from build123d import *

# Parameters (mm, degrees)
SKETCH_R     = 2.25
SKETCH_R_2   = 11.25
SKETCH_R_3   = 1.75
PAD_DEPTH    = 12
POCKET_DEPTH = 9


with BuildPart() as pocket_belt_path:
    # Sketch → Pad (new body)
    with BuildSketch(Plane.XY):
        Polygon((0, 0), (105, 0), (105, 62), (20, 62), (20, 42), (0, 42), align=None)
        with Locations((35, 10)):
            Circle(SKETCH_R, mode=Mode.SUBTRACT)
        with Locations((30, 35)):
            Circle(SKETCH_R, mode=Mode.SUBTRACT)
        with Locations((84, 21)):
            Circle(SKETCH_R_2, mode=Mode.SUBTRACT)
        with Locations((68.5, 36.5)):
            Circle(SKETCH_R_3, mode=Mode.SUBTRACT)
        with Locations((99.5, 36.5)):
            Circle(SKETCH_R_3, mode=Mode.SUBTRACT)
        with Locations((68.5, 5.5)):
            Circle(SKETCH_R_3, mode=Mode.SUBTRACT)
        with Locations((99.5, 5.5)):
            Circle(SKETCH_R_3, mode=Mode.SUBTRACT)
        with Locations((10, 30)):
            Circle(SKETCH_R, mode=Mode.SUBTRACT)
        with Locations((10, 15)):
            Circle(SKETCH_R, mode=Mode.SUBTRACT)
        with Locations((39, 52)):
            Circle(SKETCH_R, mode=Mode.SUBTRACT)
        with Locations((94, 52)):
            Circle(SKETCH_R, mode=Mode.SUBTRACT)
        with Locations((55, 5)):
            Circle(SKETCH_R, mode=Mode.SUBTRACT)
        with BuildLine():
            Line((58.75, 25), (58.75, 40))
            ThreePointArc((58.75, 40), (56.5, 42.25), (54.25, 40))
            Line((54.25, 25), (54.25, 40))
            ThreePointArc((54.25, 25), (56.5, 22.75), (58.75, 25))
        make_face(mode=Mode.SUBTRACT)
    extrude(amount=PAD_DEPTH)

    # Sketch001 → Pocket (cut)
    with BuildSketch(Plane.XY.offset(12)):
        with BuildLine():
            ThreePointArc((38.485281, 42), (36.015595, 44.209377), (32.999996, 45.583006))
            Line((32.999996, 67), (32.999996, 45.583006))
            Line((20, 67), (32.999996, 67))
            Line((20, -1), (20, 67))
            Line((20, -1), (48.252269, -1))
            Line((48.252269, 11), (48.252269, -1))
            Line((48.252269, 11), (70.252269, 11))
            ThreePointArc((70.252269, 11), (71.759618, 9.202833), (73.499996, 7.630258))
            Line((73.499996, 7.630258), (73.499996, -1))
            Line((73.499996, -1), (93.499996, -1))
            Line((93.499996, -1), (93.499996, 6.902128))
            ThreePointArc((93.499996, 6.902128), (95.574295, 8.548671), (97.367695, 10.497399))
            Line((105.499996, 10.497399), (97.367695, 10.497399))
            Line((105.499996, 30.497399), (105.499996, 10.497399))
            Line((98.099621, 30.497399), (105.499996, 30.497399))
            ThreePointArc((98.099621, 30.497399), (91.98574, 36.007594), (83.999996, 38))
            Line((83.999996, 38), (83.999996, 67))
            Line((83.999996, 67), (43.999996, 67))
            Line((43.999996, 67), (43.999996, 42))
            Line((38.485281, 42), (43.999996, 42))
        make_face()
    extrude(amount=-POCKET_DEPTH, mode=Mode.SUBTRACT)


with BuildPart() as part_mirroring:
    # Part__Mirroring: instance of Pocket belt path
    add(pocket_belt_path.part.mirror(Plane(origin=(0, 0, 0), x_dir=(0, 1, 0), z_dir=(0, 0, 1))))


solid = part_mirroring.part
Source: CAD feature listing. Evaluate the final solid. Frame: model axes, mm. A direction names the side the tool comes from. Round coordinates to 2 decimals unless told otherwise and drop trailing zeros. Loops run counter-clockwise (first coordinate to the right, second up) from the corner with the lowest first, then second, coordinate; pieces in that order, holes last. Notation, with made-up numbers: M 44.25,53.25 L 79.25,53.25 A8 cw 79.25,64.25 Z; hole C 41,40.25 d6. An arc over 180 degrees is marked long. Return JSON: item names as keys, results as strings. Group by question number.
1. Mould query, pull axis Y, two halves, no side actions, for faces 4 (the face through (94.39, 16.69, -1.48)), 5 (the face through (105, 31, -6)), 6 (the face through (73, 62, -2)). Classes: released by +Y, released by -Y, zero draft, split by the parting line, or undercut.
2. Section query B-B on x = 10. Output: boundary loops of the cut face in (y, z).
3. Section query D-D on x = 88. Output: boundary loops of the cut face in (y, z).
4. Section query C-C on y = 15. Output: boundary loops of the cut face in (x, z), and give its area (3 significant figures).
5. Pin query (flat end, axial travel): pin 1 (4.5 mm diameter, centred on y = 27, z = -7, fed in from +X); pin 2 (5 mm diameter, centred on x = 75.5, z = -10, fed in from +Y); pin 3 (0.9 mm diameter, centred on y = 50, z = -2, fed in from -X); pin 4 (2 mm diameter, centred on x = 99.5, y = 36.5, fed in from +Z). Return the tip coordinate at first contact, or that it passes through.
6. Reachability of faces 1 (the face through (33, 54, -8)), 2 (the face through (20, 21, -8)), 3 (the face through (59, 11, -8)) from +Z, -Z, +X, -X, +Y, -Y: full face, straight path, thin tool, end or side. Return the list, or none.
7. Section query A-A on z = -9. State how many separate pieces and enclosed holes the cut face has, and give its area (3 significant figures).
8. Material intervals for line 1 along Y through (x, z) = (10, -4.25); line 2 along X through (y, z) = (37, -2); line 3 along X through (y, z) = (50, -1.5), sorted ascending. Write a range as from..to.
Checks:
{
 "1": {"face 4": "undercut", "face 5": "zero draft", "face 6": "released by +Y"},
 "2": {"outline": "M 0,-12 L 12.75,-12 L 12.75,0 L 0,0 Z; M 17.25,-12 L 27.75,-12 L 27.75,0 L 17.25,0 Z; M 32.25,-12 L 42,-12 L 42,0 L 32.25,0 Z"},
 "3": {"outline": "M 0,-3 L 10.49,-3 L 10.49,0 L 0,0 Z; M 31.51,-3 L 37.52,-3 L 37.52,-12 L 62,-12 L 62,0 L 31.51,0 Z"},
 "4": {"outline": "M 0,-12 L 7.75,-12 L 7.75,0 L 0,0 Z; M 12.25,-12 L 20,-12 L 20,-3 L 74.48,-3 L 74.48,0 L 12.25,0 Z; M 93.52,-3 L 105,-3 L 105,0 L 93.52,0 Z", "area": "384 mm²"},
 "5": {"pin 1": "stops at x = 20", "pin 2": "stops at y = 8.04", "pin 3": "stops at x = 20", "pin 4": "passes through"},
 "6": {"face 1": "-Z, -X, +Y, -Y", "face 2": "-Z, +Y, -Y", "face 3": "-Z, +X, +Y"},
 "7": {"separate pieces": "5", "enclosed holes": "8", "area": "1,910 mm²"},
 "8": {"line 1": "y = 0..12.75, 17.25..27.75, 32.25..42", "line 2": "x = 0..28.97, 31.03..54.25, 58.75..66.82, 70.18..97.82, 101.18..105", "line 3": "x = 20..37.97, 40.03..92.97, 95.03..105"}
}
